from build123d import *

# Parameters (mm, degrees)
SKETCH_1_R          = 3.75
SKETCH_1_R_2        = 1.3
SKETCH_1_R_3        = 2.7
EXTRUDE_1_DEPTH     = 2.25
SKETCH_7_R          = 5.05
CUT_EXTRUDE_4_DEPTH = 4.1


with BuildPart() as part:
    # 草图1 → 凸台-拉伸1 (new body, symmetric)
    with BuildSketch(Plane.ZY):
        with BuildLine():
            Line((-4, 30), (4, 30))
            ThreePointArc((4, 30), (4.707106781, 29.707106781), (5, 29))
            Line((5, 29), (5, 8.306623863))
            ThreePointArc((5, 8.306623863), (5.297300284, 6.608208312), (6.153846154, 5.111768531))
            ThreePointArc((6.153846154, 5.111768531), (7.130688706, 3.626744901), (7.755507367, 1.962678138))
            ThreePointArc((7.755507367, 1.962678138), (8.255259703, 0.719581246), (9.067165566, -0.346181931))
            Line((9.067165566, -0.346181931), (27.451942184, -18.730958549))
            ThreePointArc((27.451942184, -18.730958549), (27.451942184, -27.216239924), (18.96666081, -27.216239924))
            Line((18.96666081, -27.216239924), (0.956494183, -9.206073297))
            ThreePointArc((0.956494183, -9.206073297), (-0.214644447, -8.335970475), (-1.587101368, -7.840989048))
            ThreePointArc((-1.587101368, -7.840989048), (-7.544802804, -2.660065909), (-6.153846154, 5.111768531))
            ThreePointArc((-6.153846154, 5.111768531), (-5.297300284, 6.608208312), (-5, 8.306623863))
            Line((-5, 8.306623863), (-5, 29))
            ThreePointArc((-5, 29), (-4.707106781, 29.707106781), (-4, 30))
        make_face()
        Circle(SKETCH_1_R, mode=Mode.SUBTRACT)
        with Locations((0, 27)):
            Circle(SKETCH_1_R_2, mode=Mode.SUBTRACT)
        with Locations((23.452077304, -23.216375043)):
            Circle(SKETCH_1_R_3, mode=Mode.SUBTRACT)
    extrude(amount=EXTRUDE_1_DEPTH, both=True)

    # 草图7 → 切除-拉伸4 (cut)
    with BuildSketch(Plane.ZY.offset(-2.25)):
        Circle(SKETCH_7_R)
    extrude(amount=CUT_EXTRUDE_4_DEPTH, mode=Mode.SUBTRACT)


solid = part.part
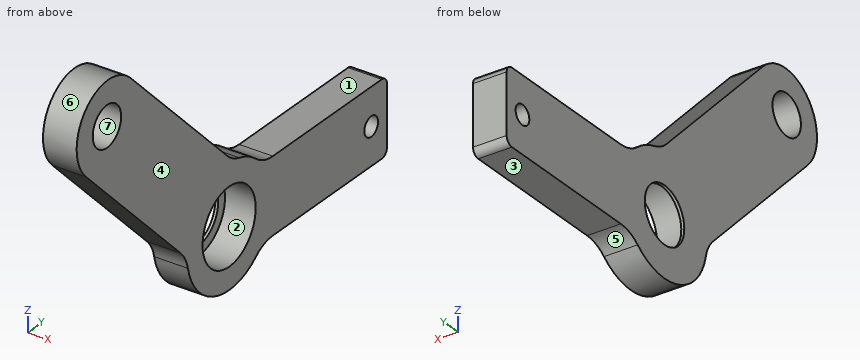
Can you work these out from the model? Positions are in its coordinate system, mm. Face numbers are marked on the shaded views. A direction names the side the tool comes from. Give positions to 0.01 mm unless a question says otherwise; leave off trailing zeros. Loops run counter-clockwise (first coordinate to the right, second up) from the corner with the lowest first, then second, coordinate; pieces in that order, holes last. Notation, with made-up numbers: M 65,9 L 105,9 A14 ccw 105,19 Z; hole C -34,-8.5 d6. An arc over 180 degrees is marked long. One line per item, written item: value. Start each with the question number.
1) If we section it at B-B, the plane z = 2: Write out the boundary of the cut face in (x, y).
2) On a 3-axis mill with a long thin cutter (end or side, diameter ignored), from which of +Z, -Z, +X, -X, +Y, -Y can I reach the whole of each face in a straight line? I mean the marked faces 1, 2, 3 and 4. Say none if no direction works.
3) If we section it at D-D, the plane y = -24: Write out the boundary of the cut face in (x, z).
4) If I drill on line 1 (Y direction, x = -0.8, z = 0); line 2 (Y direction, x = -2, z = 0); line 3 (Z direction, x = -0.4, y = -22), over which ranges is the centre line in solid material (lowest first)? Write a range as [from, to].
5) If we section it at A-A, the plane y = 27: Write out the boundary of the cut face in (x, z).
6) If we section it at C-C, the plane x = -0.2: Write out the boundary of the cut face in (y, z), and give its area (3 significant figures).
7) Thinking about a two-plate mould opening in Y: for the marked faces 5, 6 and 7, which applies, +Y half, -Y half, draft (parallel to the pull), parting line (faces both ways), or undercut?
Completed:
1. outline: M -2.25,-10.25 L 2.25,-10.25 L 2.25,-4.64 L -1.85,-4.64 L -1.85,-3.17 L -2.25,-3.17 Z; M -2.25,3.17 L -1.85,3.17 L -1.85,4.64 L 2.25,4.64 L 2.25,30 L -2.25,30 Z
2. face 1: +Z, +X, -X, +Y
2. face 2: +X
2. face 3: -Z, +X, -X, +Y
2. face 4: +Z, -Z, +X, +Y, -Y
3. outline: M -2.25,15.75 L 2.25,15.75 L 2.25,20.87 L -2.25,20.87 Z; M -2.25,26.04 L 2.25,26.04 L 2.25,29.12 L -2.25,29.12 Z
4. line 1: y = [-8.46, -5.05], [5.05, 25.7], [28.3, 30]
4. line 2: y = [-8.46, -3.75], [3.75, 25.7], [28.3, 30]
4. line 3: z = [13.75, 21.04], [25.86, 29.13]
5. outline: M -2.25,-5 L 2.25,-5 L 2.25,-1.3 L -2.25,-1.3 Z; M -2.25,1.3 L 2.25,1.3 L 2.25,5 L -2.25,5 Z
6. outline: M -27.22,18.97 L -9.21,0.96 A5 cw -7.84,-1.59 A8 ccw 5.11,-6.15 A5 cw 8.31,-5 L 29,-5 A1 ccw 30,-4 L 30,4 A1 ccw 29,5 L 8.31,5 A5 cw 5.11,6.15 A8 ccw 1.96,7.76 A5 cw -0.35,9.07 L -18.73,27.45 A6 ccw Z; hole C -23.22,23.45 d5.4; hole C 0,0 d10.1; hole C 27,0 d2.6
6. area: 682 mm^2
7. face 5: +Y half
7. face 6: parting line
7. face 7: undercut
